from build123d import *

# Parameters (mm, degrees)
F0_W     = 55.88
F0_H     = 15.875
F1_DEPTH = 9.525
F2_D     = 5.1054
F3_D     = 9.525


with BuildPart() as f1:
    # F0 (on Top) → F1 (new body)
    with BuildSketch(Plane.XY):
        Rectangle(F0_W, F0_H)
    extrude(amount=F1_DEPTH)

    # F2 (through all)
    with Locations(Plane(origin=(0, 0, 0), x_dir=(1, 0, 0), z_dir=(0, 0, -1))):
        with Locations((-23.9776, 0), (23.9776, 0)):
            Hole(F2_D / 2)

    # F3 (through all)
    with Locations(Plane(origin=(0, 0, 0), x_dir=(1, 0, 0), z_dir=(0, 0, -1))):
        with Locations((0, 0)):
            Hole(F3_D / 2)


solid = f1.part
Input: part model. Units: mm. Frame: model coordinates. Round coordinates to 2 decimals unless told otherwise and drop trailing zeros. Order: outer loops, then holes, each group sorted by start corner. A loop starts at its lowest first (then second) coordinate and runs counter-clockwise, first axis right, second up. Notation, with made-up numbers: (64.25, -37.75) - (98.25, -37.75) arc R30 ccw to (98.25, -11.75) - close; hole circle Ø4 at (9.5, -30). An arc over 180 degrees is marked (long way). Answer as a JSON object with one key per item and string values. Group by question number.
(1) Draft query along X for faces 1 (the face through (3.78, 2.9, 4.83)), 2 (the face through (27.94, 0, 5)), 3 (the face through (0, -5, 0)). Return one class per face: released by +X, released by -X, zero draft, split by the parting line, or undercut.
(2) Cut plane C-C (z = 5.25). Return loops of the section in (x, y) (1 decimal), then the cut area to 3 significant figures.
(3) Cut plane A-A (x = 0). Return loops of the section in (y, z) (1 decimal), then the cut area to 3 significant figures.
(4) Material intervals for probe 1 along Y at (x, z) = (0, 7.5); probe 2 along X at (y, z) = (1.5, 7.25); probe 3 along X at (y, z) = (4, 6.25), sorted ascending. Write a range as from..to.
(5) Cut plane D-D (x = -22). Return loops of the section in (y, z) (1 decimal).
(6) Cut plane B-B (y = 0). Return loops of the section in (x, z) (1 decimal).
Here are the results:
{
 "1": {"face 1": "undercut", "face 2": "released by +X", "face 3": "zero draft"},
 "2": {"outline": "(-27.9, -7.9) - (27.9, -7.9) - (27.9, 7.9) - (-27.9, 7.9) - close; hole circle Ø5.1 at (-24, 0); hole circle Ø9.5 at (0, 0); hole circle Ø5.1 at (24, 0)", "area": "775 mm^2"},
 "3": {"outline": "(-7.9, 0) - (-4.8, 0) - (-4.8, 9.5) - (-7.9, 9.5) - close; (4.8, 0) - (7.9, 0) - (7.9, 9.5) - (4.8, 9.5) - close", "area": "60.5 mm^2"},
 "4": {"probe 1": "y = -7.94..-4.76, 4.76..7.94", "probe 2": "x = -27.94..-26.04, -21.91..-4.52, 4.52..21.91, 26.04..27.94", "probe 3": "x = -27.94..-2.58, 2.58..27.94"},
 "5": {"outline": "(-7.9, 0) - (-1.6, 0) - (-1.6, 9.5) - (-7.9, 9.5) - close; (1.6, 0) - (7.9, 0) - (7.9, 9.5) - (1.6, 9.5) - close"},
 "6": {"outline": "(-27.9, 0) - (-26.5, 0) - (-26.5, 9.5) - (-27.9, 9.5) - close; (-21.4, 0) - (-4.8, 0) - (-4.8, 9.5) - (-21.4, 9.5) - close; (4.8, 0) - (21.4, 0) - (21.4, 9.5) - (4.8, 9.5) - close; (26.5, 0) - (27.9, 0) - (27.9, 9.5) - (26.5, 9.5) - close"}
}
